Study the drawing (mm; zero at the part's minimum x, y, z) and answer. A direction names the side the tool comes from. Round coordinates to 2 decimals unless told otherwise and drop trailing zeros. Loops run counter-clockwise (first coordinate to the right, second up) from the corner with the lowest first, then second, coordinate; pieces in that order, holes last. Notation, with made-up numbers: M 16.5,3 L 58.5,3 A18 cw 58.5,18 Z; hole C 89,86.5 d1. An arc over 180 degrees is marked long. Put each result on its own line as item: value. Start each with the question number.
(1) Section B-B, the plane x = 37 is taken. Determine the outline of the cut face in (y, z), then the cut area to 4 significant figures.
(2) Which of the six approach directions +Z, -Z, +X, -X, +Y, -Y give full straight-line access (tool end or side, diameter ignored) to the marked faces 5, 6, 7, 8 and 9?
(3) Flat-ended cylindrical pins translate along their axes: P1, Ø6, axis at y = 18.5, z = 6.5, coming from the -X side; P2, Ø2, axis at y = 37.5, z = 10.5, coming from the -X side; P3, Ø1.5, axis at y = 23, z = 4, coming from the +X side. Find the tip coordinate at first contact, or state that the pin passes through.
(4) Determine the mould class of the marked faces 1, 2, 3 and 4 for opening direction Z: released by +Z, released by -Z, zero draft, split by the parting line, or undercut.
(5) Section D-D, the plane x = 67 is taken. Determine the outline of the cut face in (y, z), then the cut area to 3 significant figures.
(6) Section C-C, the plane y = 28.5 is taken. Determine the outline of the cut face in (x, z), then the cut area to 3 significant figures.
(7) Straight lines are drawn through the part: line 1 (X direction, y = 5.75, z = 6); line 2 (Y direction, x = 37, z = 2.65); line 3 (Y direction, x = 37, z = 7.5). For each, find the intervals that lie inside material, in ascending order.
(8) Section A-A, the plane z = 6 is taken. Determine the outline of the cut face in (x, y), then the cut area to 3 significant figures.
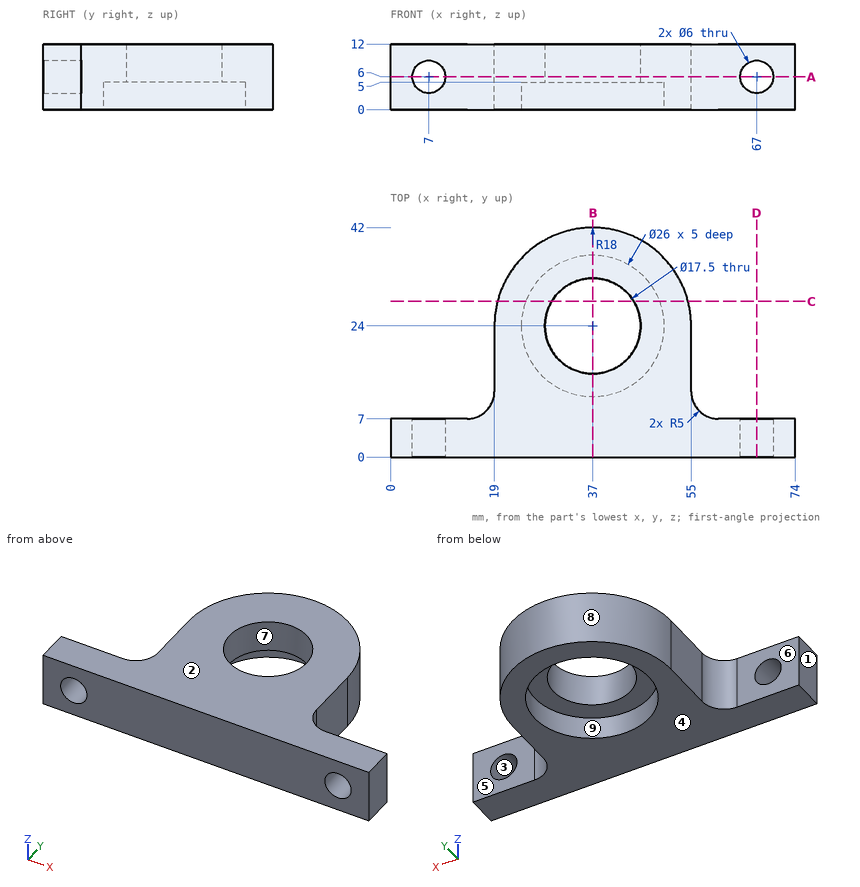
Recorded:
1. outline: M 0,0 L 11,0 L 11,5 L 15.25,5 L 15.25,12 L 0,12 Z; M 32.75,5 L 37,5 L 37,0 L 42,0 L 42,12 L 32.75,12 Z
1. area: 251.5 mm²
2. face 5: +Z, -Z, +X, +Y
2. face 6: +Z, -Z, -X, +Y
2. face 7: +Z, -Z
2. face 8: +Z, -Z, +Y
2. face 9: -Z
3. P1: stops at x = 19
3. P2: stops at x = 24.05
3. P3: stops at x = 55
4. face 1: zero draft
4. face 2: released by +Z
4. face 3: undercut
4. face 4: released by -Z
5. outline: M 0,0 L 7,0 L 7,3 L 0,3 Z; M 0,9 L 7,9 L 7,12 L 0,12 Z
5. area: 42.0 mm²
6. outline: M 19.57,0 L 24.8,0 L 24.8,5 L 29.5,5 L 29.5,12 L 19.57,12 Z; M 44.5,5 L 49.2,5 L 49.2,0 L 54.43,0 L 54.43,12 L 44.5,12 Z
6. area: 191 mm²
7. line 1: x = 0 to 4, 10 to 64, 70 to 74
7. line 2: y = 0 to 11, 37 to 42
7. line 3: y = 0 to 15.25, 32.75 to 42
8. outline: M 0,0 L 4,0 L 4,7 L 0,7 Z; M 10,0 L 64,0 L 64,7 L 60,7 A5 cw 55,12 L 55,24 A18 ccw 19,24 L 19,12 A5 cw 14,7 L 10,7 Z; M 70,0 L 74,0 L 74,7 L 70,7 Z; hole C 37,24 d17.5
8. area: 1,330 mm²
